Autodesk Inventor part; units mm, degrees
ref_plane "YZ Plane" through (0, 0, 0) normal (1, 0, 0) x (0, 1, 0)
ref_plane "XZ Plane" through (0, 0, 0) normal (0, 1, 0) x (-1, 0, 0)
ref_plane "XY Plane" through (0, 0, 0) normal (0, 0, 1) x (1, 0, 0)
sketch "Sketch1" plane through (0, 0, 0) normal (0, 1, 0) x (-1, 0, 0)
  line L0 (0, 0) -> (100, 0)
  line L1 (100, 0) -> (100, -60)
  line L2 (100, -60) -> (0, -60)
  line L3 (0, -60) -> (0, 0)
  line L4 (100, -52.4106) -> (95, -52.4106) construction
  line L5 (100, -52.4106) -> (105, -52.4106) construction
  line L6 (95, -60) -> (95, -55)
  line L7 (95, -55) -> (22, -55)
  line L8 (22, -55) -> (22, -15)
  line L9 (22, -15) -> (95, -15)
  line L10 (95, -15) -> (95, -55)
  line L11 (100, 0) -> (0, -60) construction
  line L12 (100, -60) -> (0, 0) construction
  line L13 (-5, -65) -> (105, -65)
  line L14 (105, -65) -> (105, 5)
  line L15 (105, 5) -> (-5, 5)
  line L16 (-5, 5) -> (-5, -65)
  line L17 (-5, -65) -> (105, 5) construction
  line L18 (105, -65) -> (-5, 5) construction
  line L19 (95, -15) -> (22, -55) construction
  line L20 (95, -55) -> (22, -15) construction
  line L21 (20.5, -13) -> (96.5, -13)
  line L22 (96.5, -13) -> (96.5, -57)
  line L23 (96.5, -57) -> (20.5, -57)
  line L24 (20.5, -57) -> (20.5, -13)
  line L25 (20.5, -13) -> (96.5, -57) construction
  line L26 (96.5, -13) -> (20.5, -57) construction
  point P0 (50, -30)
  point P1 (58.5, -35)
  dimension "d0" = 100
  dimension "d1" = 60
  dimension "d2" = 5
  dimension "d3" = 180
  dimension "d4" = 5
  dimension "d5" = 73
  dimension "d6" = 40
  dimension "d7" = 110
  dimension "d8" = 70
  dimension "d9" = 76
  dimension "d10" = 44
extrude "Extrusion1" add sketch "Sketch1" along normal blind 30 contours L16 L15 L14 L13
extrude "Extrusion2" add sketch "Sketch1" along normal blind 22 contours L21 L22 L23 L24
extrude "Extrusion3" add sketch "Sketch1" along normal blind 2.5 contours L0 L1 L2 L3
sketch "Sketch2" plane through (0, 22, 0) normal (0, 1, 0) x (1, 0, 0)
  line L0 (-20.5, 57) -> (-96.5, 57)
  line L1 (-96.5, 13) -> (-20.5, 13)
  line L2 (-96.5, 57) -> (-20.5, 57)
  line L3 (-20.5, 57) -> (-20.5, 13)
  line L4 (-20.5, 13) -> (-96.5, 13)
  line L5 (-96.5, 13) -> (-96.5, 57)
  point P0 (0, 0)
extrude "Extrusion4" add sketch "Sketch2" along normal blind 2.5
sketch "Sketch4" plane through (-20.5, 2.5, -13) normal (1, 0, 0) x (0, 0, -1)
  line L0 (-18, -2.5) -> (-18, 27.5)
  line L1 (-18, 27.5) -> (-13, 27.5)
  line L2 (-13, 27.5) -> (-13, 0)
  line L3 (-13, 0) -> (0, 0)
  line L4 (0, 0) -> (44, 0)
  line L5 (44, 0) -> (47, 0)
  line L6 (47, 0) -> (47, 27.5)
  line L7 (47, 27.5) -> (52, 27.5)
  line L8 (52, 27.5) -> (52, -2.5)
  line L9 (52, -2.5) -> (-18, -2.5)
  line L10 (0, 0) -> (0, 22)
  line L11 (0, 22) -> (44, 22)
  line L12 (44, 22) -> (44, 0)
  line L13 (0, 22) -> (44, 22)
  line L14 (44, 22) -> (0, 22)
  line L15 (-18, -2.5) -> (52, -2.5)
  line L16 (52, -2.5) -> (52, 27.5)
  line L17 (-18, 27.5) -> (52, 27.5)
  line L18 (-18, -2.5) -> (-18, 27.5)
  line L19 (0, 0) -> (44, 0)
  line L20 (44, 0) -> (44, 22)
  line L21 (0, 22) -> (44, 22)
  line L22 (0, 0) -> (0, 22)
  line L23 (44, 0) -> (44, 22) construction
  line L24 (44, 22) -> (0, 0) construction
  line L25 (44, 0) -> (0, 0) construction
  line L26 (44, 22) -> (0, 22) construction
  line L27 (44, 0) -> (0, 22) construction
  line L28 (27, 8.5) -> (17, 8.5)
  line L29 (17, 8.5) -> (17, 13.5)
  line L30 (17, 13.5) -> (27, 13.5)
  line L31 (27, 13.5) -> (27, 8.5)
  line L32 (27, 8.5) -> (17, 13.5) construction
  line L33 (17, 8.5) -> (27, 13.5) construction
  point P0 (-13, -2.5)
  point P1 (22, 11)
  dimension "d19" = 10
  dimension "d20" = 5
extrude "Extrusion5" cut sketch "Sketch4" against normal blind 10 contours L28 L29 L30 L31
fillet "Fillet1" radius 2 8 edges at (-58.5, 24.5, -57) (-20.5, 24.5, -35) (-58.5, 24.5, -13) (-96.5, 24.5, -35) (-20.5, 13.5, -13) (-20.5, 13.5, -57) (-96.5, 13.5, -13) (-96.5, 13.5, -57)
sketch "Sketch5" plane through (0, 22, 0) normal (0, -1, 0) x (1, 0, 0)
  line L0 (-22, -55) -> (-22, -15) construction
  line L1 (-94.5, -55) -> (-96.5, -55) construction
  line L2 (-58.5, -35) -> (-58.5, -55) construction
  line L3 (-58.5, -55) -> (-58.5, -45) construction
  line L4 (-58.5, -15) -> (-58.5, -25) construction
  point P0 (0, 0)
  dimension "d24" = 10
  dimension "d25" = 10
hole "Hole1" at (-58.5, 22, -45) at (-58.5, 22, -25) direction (0, 1, 0) diameter 1.5 depth 40 tip angle 118
sketch "Sketch6" plane through (0, 24.5, 0) normal (0, 1, 0) x (1, 0, 0)
  circle A0 centre (-58.5, 45) radius 0.75
  circle A1 centre (-58.5, 45) radius 2
  circle A2 centre (-58.5, 25) radius 0.75
  circle A3 centre (-58.5, 25) radius 2
  point P0 (0, 0)
  dimension "d33" = 4
  dimension "d34" = 4
extrude "Extrusion6" cut sketch "Sketch6" against normal blind 1.5
fillet "Fillet2" radius 2 4 edges at (-50, 0, -65) (-105, 0, -30) (-50, 0, 5) (5, 0, -30)
sketch "Sketch7" plane through (0, 30, 0) normal (0, 1, 0) x (1, 0, 0)
  line L0 (0, 60) -> (2.5, 60)
  line L1 (2.5, 60) -> (2.5, 0)
  line L2 (2.5, 0) -> (0, 0)
  line L3 (0, 0) -> (0, 60)
  dimension "d46" = 2.5
extrude "Extrusion7" cut sketch "Sketch7" against normal blind 27.5
fillet "Fillet3" radius 2 8 edges at (-104.4142, 0.5858, 4.4142) (-105, 16, 5) (4.4142, 0.5858, 4.4142) (5, 16, 5) (-104.4142, 0.5858, -64.4142) (-105, 16, -65) (4.4142, 0.5858, -64.4142) (5, 16, -65)
properties part number "abajo model2"
The listing builds one solid part. Answer for the finished solid, in the listing's coordinates (mm). A direction names the side the tool comes from. Round coordinates to 2 decimals unless told otherwise and drop trailing zeros. Loops run counter-clockwise (first coordinate to the right, second up) from the corner with the lowest first, then second, coordinate; pieces in that order, holes last. Notation, with made-up numbers: (4, 28.5) - (10, 28.5) arc R37 ccw to (10, 67.5) - close; hole circle Ø11 at (-25, 61.5). An arc over 180 degrees is marked (long way). Use one line per item in the form item = value. Start each with the question number.
1. The part is cut by section B-B on z = -36. Determine the outline of the cut face in (x, y).
2. The part is cut by section C-C on y = 8. Determine the outline of the cut face in (x, z).
3. The part is cut by section A-A on y = 27. Determine the outline of the cut face in (x, z).
4. The part is cut by section D-D on x = -73.5. Determine the outline of the cut face in (y, z), then the cut area to 3 significant figures.
5. Consider line 1 (Z direction, x = -91, y = 13); line 2 (X direction, y = 22.5, z = -45); line 3 (Z direction, x = -58.5, y = 22.3). Determine where each line is inside the solid, lowest interval first. Write a range as [from, to].
6. A tool of negligible diameter and unlimited length cuts with its end or side. For faces 1 (the face through (-58, 12, -57)), 2 (the face through (-49, 16, -65)), 3 (the face through (-95, 11, -35)), from which of +Z, -Z, +X, -X, +Y, -Y can it reach the whole face along a straight path? Write none if from no direction.
7. Given pin 1 Ø3 at (x, z) = (-58.5, -25) entering from +Y; pin 2 Ø3 at (x, z) = (-58.5, -45) entering from -Y; pin 3 Ø1.5 at (x, z) = (-77, -50.5) entering from +Y, each flat-ended and moving along its own axis, determine where each tip first touches the part or whether it passes through.
Geometry check:
q1.outline = (-105, 2) arc R2 ccw to (-103, 0) - (-95, 0) - (-95, 22) - (-22, 22) - (-22, 16) - (-20.5, 16) - (-20.5, 22.5) arc R2 ccw to (-22.5, 24.5) - (-94.5, 24.5) arc R2 ccw to (-96.5, 22.5) - (-96.5, 2.5) - (-100, 2.5) - (-100, 30) - (-105, 30) - close; (-22, 0) - (3, 0) arc R2 ccw to (5, 2) - (5, 30) - (2.5, 30) - (2.5, 2.5) - (-20.5, 2.5) - (-20.5, 11) - (-22, 11) - close
q2.outline = (-105, -63) arc R2 ccw to (-103, -65) - (3, -65) arc R2 ccw to (5, -63) - (5, 3) arc R2 ccw to (3, 5) - (-103, 5) arc R2 ccw to (-105, 3) - close; (-96.5, -55) arc R2 ccw to (-94.5, -57) - (-22.5, -57) arc R2 ccw to (-20.5, -55) - (-20.5, -15) arc R2 ccw to (-22.5, -13) - (-94.5, -13) arc R2 ccw to (-96.5, -15) - close; hole (-100, -60) - (2.5, -60) - (2.5, 0) - (-100, 0) - close; hole (-95, -55) - (-22, -55) - (-22, -15) - (-95, -15) - close
q3.outline = (-105, -63) arc R2 ccw to (-103, -65) - (3, -65) arc R2 ccw to (5, -63) - (5, 3) arc R2 ccw to (3, 5) - (-103, 5) arc R2 ccw to (-105, 3) - close; hole (-100, -60) - (2.5, -60) - (2.5, 0) - (-100, 0) - close
q4.outline = (0, -63) arc R2 ccw to (2, -65) - (30, -65) - (30, -60) - (2.5, -60) - (2.5, -57) - (22.5, -57) arc R2 ccw to (24.5, -55) - (24.5, -15) arc R2 ccw to (22.5, -13) - (2.5, -13) - (2.5, 0) - (30, 0) - (30, 5) - (2, 5) arc R2 ccw to (0, 3) - (0, -15) - (22, -15) - (22, -55) - (0, -55) - close
q4.area = 535 mm^2
q5.line_1 = [-65, -60], [-57, -55], [-15, -13], [0, 5]
q5.line_2 = [-105, -100], [-96.5, -59.25], [-57.75, -20.5], [2.5, 5]
q5.line_3 = [-65, -60], [-57, -45.75], [-44.25, -25.75], [-24.25, -13], [0, 5]
q6.face_1 = +Y
q6.face_2 = -Z, +X, -X, +Y, -Y
q6.face_3 = -Y
q7.pin_1 = 23
q7.pin_2 = 22
q7.pin_3 = 24.5
